Here's how the part is built. I have some questions about the finished solid (model axes, mm). Face numbers are marked on the shaded views. A direction names the side the tool comes from. Round coordinates to 2 decimals unless told otherwise and drop trailing zeros. Write each loop counter-clockwise with the first axis right and the second up, starting at its lowest first coordinate (ties: lowest second). Pieces come first, ordered by that corner, then holes. Notation, with made-up numbers: (49.5, -8.5) - (86.5, -8.5) arc R10 ccw to (86.5, -1.5) - close; hole circle Ø9 at (-9, 88.25). An arc over 180 degrees is marked (long way). One line per question, with ' | ' between items. Start each with the question number.
(1) For the marked faces 5, 6, 7 and 8, which set-ups out of +Z, -Z, +X, -X, +Y, -Y let a thin tool reach every point of the face, with its end or its side?
(2) Thinking about a two-plate mould opening in X: for the marked faces 1, 2, 3 and 4, which applies, pulls with the +X half, pulls with the -X half, needs draft (parallel to the pull), parting line crosses it, or undercut?
(3) Imagine slicing it at D-D (x = -0.5). Give the number of separate pieces and of enclosed holes in the cut face, plus the area to 3 significant figures.
(4) Imagine slicing it at A-A (x = -2.5). Write out the boundary of the cut face in (y, z).
(5) Will these pins go through, and if not, where does the flat tip stop? pin 1 (10 mm diameter, centred on x = -5, y = 0, fed in from -Z); pin 2 (1.1 mm diameter, centred on x = 0.5, z = -0.5, fed in from +Y); pin 3 (4 mm diameter, centred on x = -2, z = 16, fed in from -Y).
(6) If I drill on L1, parallel to X at y = -0.5, z = 10.75; L2, parallel to Y at x = 4, z = 5.75; L3, parallel to Z at x = -2.5, y = -6.75, over which ranges is the centre line in solid material (lowest first)?
(7) Imagine slicing it at B-B (y = -5.25). Write out the boundary of the cut face in (x, z).
(8) Imagine slicing it at C-C (z = 6.25). Write out the boundary of the cut face in (x, y).
from build123d import *

# Parameters (mm, degrees)
SKETCH_1_W          = 17
SKETCH_1_H          = 20
EXTRUDE_1_DEPTH     = 3
SKETCH_2_W          = 17
SKETCH_2_H          = 3
EXTRUDE_2_DEPTH     = 17
EXTRUDE_3_DEPTH     = 2
EXTRUDE_4_DEPTH     = 2
EXTRUDE_5_DEPTH     = 1
EXTRUDE_6_DEPTH     = 1
CUT_EXTRUDE_3_DEPTH = 21
CUT_EXTRUDE_4_DEPTH = 21


with BuildPart() as part:
    # 草图1 → 凸台-拉伸1 (new body)
    with BuildSketch(Plane.XY):
        Rectangle(SKETCH_1_W, SKETCH_1_H)
    extrude(amount=EXTRUDE_1_DEPTH)

    # 草图2 → 凸台-拉伸2 (add)
    with BuildSketch(Plane.XY.offset(3)):
        with Locations((0, 8.5)):
            Rectangle(SKETCH_2_W, SKETCH_2_H)
    extrude(amount=EXTRUDE_2_DEPTH)

    # 草图3 → 凸台-拉伸3 (add)
    with BuildSketch(Plane.ZY.offset(8.5)):
        Polygon((20, 7), (3, -10), (3, 7), align=None)
    extrude(amount=-EXTRUDE_3_DEPTH)

    # 草图4 → 凸台-拉伸4 (add)
    with BuildSketch(Plane(origin=(8.5, 0, 0), x_dir=(0, 0, -1), z_dir=(1, 0, 0))):
        Polygon((-20, 7), (-3, -10), (-3, 7), align=None)
    extrude(amount=-EXTRUDE_4_DEPTH)

    # 草图5 → 凸台-拉伸5 (add)
    with BuildSketch(Plane(origin=(0, 10, 0), x_dir=(1, 0, 0), z_dir=(0, 1, 0))):
        with BuildLine():
            Line((-1.5, -2.5), (1.5, -2.5))
            ThreePointArc((1.5, -2.5), (2, -3), (1.5, -3.5))
            Line((1.5, -3.5), (-1.5, -3.5))
            ThreePointArc((-1.5, -3.5), (-2, -3), (-1.5, -2.5))
        make_face()
        with BuildLine():
            Line((-1.5, -17), (1.5, -17))
            ThreePointArc((1.5, -17), (2, -17.5), (1.5, -18))
            Line((1.5, -18), (-1.5, -18))
            ThreePointArc((-1.5, -18), (-2, -17.5), (-1.5, -17))
        make_face()
    extrude(amount=EXTRUDE_5_DEPTH)

    # 草图6 → 凸台-拉伸6 (add)
    with BuildSketch(Plane(origin=(0, 0, 0), x_dir=(-1, 0, 0), z_dir=(0, 0, -1))):
        with BuildLine():
            Line((-1.5, 7.5), (1.5, 7.5))
            ThreePointArc((1.5, 7.5), (2, 7), (1.5, 6.5))
            Line((1.5, 6.5), (-1.5, 6.5))
            ThreePointArc((-1.5, 6.5), (-2, 7), (-1.5, 7.5))
        make_face()
        with BuildLine():
            Line((-1.5, -7), (1.5, -7))
            ThreePointArc((1.5, -7), (2, -7.5), (1.5, -8))
            Line((1.5, -8), (-1.5, -8))
            ThreePointArc((-1.5, -8), (-2, -7.5), (-1.5, -7))
        make_face()
    extrude(amount=EXTRUDE_6_DEPTH)

    # 草图7 → 切除-拉伸3 (cut, through all)
    with BuildSketch(Plane(origin=(0, 0, 0), x_dir=(-1, 0, 0), z_dir=(0, 0, -1))):
        with BuildLine():
            Line((2.95, 1.15), (2.95, -1.75))
            ThreePointArc((2.95, -1.75), (0, -4.7), (-2.95, -1.75))
            Line((-2.95, -1.75), (-2.95, 1.15))
            ThreePointArc((-2.95, 1.15), (0, 4.1), (2.95, 1.15))
        make_face()
    extrude(amount=-CUT_EXTRUDE_3_DEPTH, mode=Mode.SUBTRACT)

    # 草图8 → 切除-拉伸4 (cut, through all)
    with BuildSketch(Plane(origin=(0, 10, 0), x_dir=(1, 0, 0), z_dir=(0, 1, 0))):
        with BuildLine():
            Line((2.95, -8.85), (2.95, -11.75))
            ThreePointArc((2.95, -11.75), (0, -14.7), (-2.95, -11.75))
            Line((-2.95, -11.75), (-2.95, -8.85))
            ThreePointArc((-2.95, -8.85), (0, -5.9), (2.95, -8.85))
        make_face()
    extrude(amount=-CUT_EXTRUDE_4_DEPTH, mode=Mode.SUBTRACT)


solid = part.part
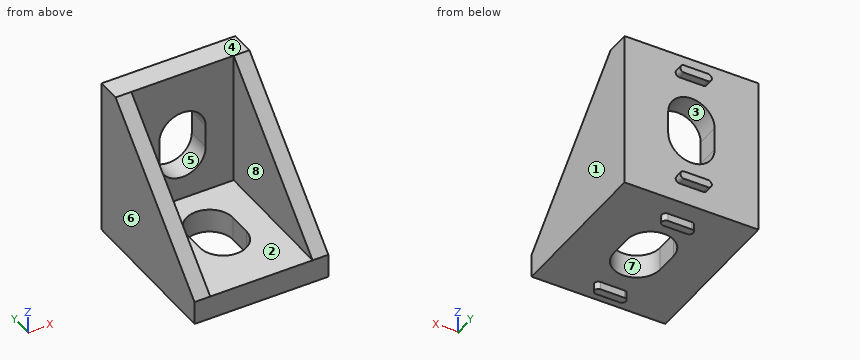
Check sheet entries:
1) face 5: +Y, -Y | face 6: +Z, -Z, -X, +Y, -Y | face 7: +Z, -Z | face 8: +Z, -Y
2) face 1: pulls with the +X half | face 2: undercut | face 3: undercut | face 4: needs draft
3) separate pieces: 3 | enclosed holes: 0 | area: 62.7 mm^2
4) outline: (-10, 0) - (-3.32, 0) - (-3.32, 3) - (-10, 3) - close; (2.72, 0) - (10, 0) - (10, 7.28) - (7, 7.28) - (7, 3) - (2.72, 3) - close; (7, 13.32) - (10, 13.32) - (10, 20) - (7, 20) - close
5) pin 1: z = 0 | pin 2: y = 10 | pin 3: y = 7
6) L1: -8.5 to -6.5, 6.5 to 8.5 | L2: 7 to 10 | L3: 0 to 3
7) outline: (-8.5, 0) - (8.5, 0) - (8.5, 7.75) - (6.5, 7.75) - (6.5, 3) - (-6.5, 3) - (-6.5, 7.75) - (-8.5, 7.75) - close
8) outline: (-8.5, -6.75) - (-6.5, -6.75) - (-6.5, 7) - (-1.39, 7) - (-1.39, 10) - (-8.5, 10) - close; (1.39, 7) - (6.5, 7) - (6.5, -6.75) - (8.5, -6.75) - (8.5, 10) - (1.39, 10) - close
